Autodesk Inventor part; units mm, degrees
ref_plane "YZ Plane" through (0, 0, 0) normal (1, 0, 0) x (0, 1, 0)
ref_plane "XZ Plane" through (0, 0, 0) normal (0, 1, 0) x (-1, 0, 0)
ref_plane "XY Plane" through (0, 0, 0) normal (0, 0, 1) x (1, 0, 0)
sketch "Sketch1" plane through (0, 0, 0) normal (0, 0, 1) x (1, 0, 0)
  line L0 (0, 0) -> (25.4, 0)
  line L1 (25.4, 0) -> (25.4, 25.4)
  line L2 (25.4, 25.4) -> (0, 25.4)
  line L3 (0, 25.4) -> (0, 0)
  line L4 (1.5875, 23.8125) -> (23.8125, 23.8125)
  line L5 (23.8125, 23.8125) -> (23.8125, 1.5875)
  line L6 (23.8125, 1.5875) -> (1.5875, 1.5875)
  line L7 (1.5875, 1.5875) -> (1.5875, 23.8125)
  dimension "d0" = 25.4
  dimension "d1" = 25.4
  dimension "d2" = 1.5875
extrude "Extrusion1" add sketch "Sketch1" against normal blind 355.6
sketch "Sketch2" plane through (0, 25.4, 0) normal (0, 1, 0) x (1, 0, 0)
  line L0 (25.4, 355.6) -> (0, 355.6)
  line L1 (0, 0) -> (0, 355.6)
  line L2 (25.4, 0) -> (0, 0)
  point P0 (12.7, 12.7)
  point P1 (12.7, 342.9)
  dimension "d5" = 12.7
  dimension "d6" = 12.7
  dimension "d7" = 12.7
hole "Hole1" at (12.7, 25.4, -12.7) at (12.7, 25.4, -342.9) direction (0, -1, 0) diameter 6.35 depth 25.4 tip angle 118
properties part number "tube_m_r_in_mid"
Can you work these out from the model? Positions are in its coordinate system, mm. A direction names the side the tool comes from. Give positions to 0.01 mm unless a question says otherwise; leave off trailing zeros. Loops run counter-clockwise (first coordinate to the right, second up) from the corner with the lowest first, then second, coordinate; pieces in that order, holes last. Notation, with made-up numbers: M 44,76.25 L 71,76.25 A23 cw 71,103.25 Z; hole C 46,-1.75 d10. An arc over 180 degrees is marked long. One line per item, written item: value. Start each with the question number.
1) On a 3-axis mill with a long thin cutter (end or side, diameter ignored), from which of +Z, -Z, +X, -X, +Y, -Y can I reach the whole of each face in a straight line? I mean faces 1 (the face through (15.5, 0.8, -11.2)), 2 (the face through (13, 1.588, -175)). Say none if no direction works.
2) If we section it at A-A, the plane y = 20: Write out the boundary of the cut face in (x, z), and give its area (3 significant figures).
3) If we section it at D-D, the plane z = -277.5: Write out the boundary of the cut face in (x, y).
4) If I drill on line 1 (Z direction, x = 12.7, y = 24.6) (3 decimals); line 2 (X direction, y = 24.4, z = -342.9) (3 decimals); line 3 (X direction, y = 10.75, z = -68.5), over which ranges is the centre line in solid material (lowest first)? Write a range as [from, to].
5) If we section it at C-C, the plane x = 12.7: Write out the boundary of the cut face in (y, z) (1 decimal), and give its area (3 significant figures).
6) I'm going to push a flat-ended pin straight in: pin 1 (5 mm diameter, centred on x = 12.7, z = -12.7, fed in from +Y). Where does the tip first touch, or does it pass through?
7) Thinking about a two-plate mould opening in X: for faces 3 (the face through (0, 13, -175)), 4 (the face through (13, 23.812, -175)), 5 (the face through (1, 13, -355.6)), which applies, +X half, -X half, draft (parallel to the pull), parting line (faces both ways), or undercut?
8) If we section it at B-B, the plane z = -12.7: Write out the boundary of the cut face in (x, y) (1 decimal), and give its area (3 significant figures).
Completed:
1. face 1: +Y, -Y
1. face 2: +Z, -Z
2. outline: M 0,-355.6 L 1.59,-355.6 L 1.59,0 L 0,0 Z; M 23.81,-355.6 L 25.4,-355.6 L 25.4,0 L 23.81,0 Z
2. area: 1,130 mm^2
3. outline: M 0,0 L 25.4,0 L 25.4,25.4 L 0,25.4 Z; hole M 1.59,1.59 L 23.81,1.59 L 23.81,23.81 L 1.59,23.81 Z
4. line 1: z = [-355.6, -346.075], [-339.725, -15.875], [-9.525, 0]
4. line 2: x = [0, 9.525], [15.875, 25.4]
4. line 3: x = [0, 1.59], [23.81, 25.4]
5. outline: M 0,-355.6 L 1.6,-355.6 L 1.6,-346.1 L 0,-346.1 Z; M 0,-339.7 L 1.6,-339.7 L 1.6,-15.9 L 0,-15.9 Z; M 0,-9.5 L 1.6,-9.5 L 1.6,0 L 0,0 Z; M 23.8,-355.6 L 25.4,-355.6 L 25.4,-346.1 L 23.8,-346.1 Z; M 23.8,-339.7 L 25.4,-339.7 L 25.4,-15.9 L 23.8,-15.9 Z; M 23.8,-9.5 L 25.4,-9.5 L 25.4,0 L 23.8,0 Z
5. area: 1,090 mm^2
6. pin 1: passes through
7. face 3: -X half
7. face 4: undercut
7. face 5: draft
8. outline: M 0,0 L 9.5,0 L 9.5,1.6 L 1.6,1.6 L 1.6,23.8 L 9.5,23.8 L 9.5,25.4 L 0,25.4 Z; M 15.9,0 L 25.4,0 L 25.4,25.4 L 15.9,25.4 L 15.9,23.8 L 23.8,23.8 L 23.8,1.6 L 15.9,1.6 Z
8. area: 131 mm^2
